from build123d import *

# Parameters (mm, degrees)
SKETCH3_W         = 2.032
SKETCH3_H         = 5.588
EXTRUDE1_DEPTH    = 2.088262662
CIRPATTERN1_COUNT = 6


with BuildPart() as part:
    # Sketch2 → Revolve1 (revolve)
    with BuildSketch(Plane.XY):
        Polygon((-4, 1.088262662), (-5.8419953, 0.40140039), (-7.003246048, 0.951561432), (-7.257246048, 0.951561432), (-7.3659953, 0.722019279), (-5.8419953, 0), (-4, 0.686862271), align=None)
    revolve(axis=Axis((0, 0, 0), (0, 1, 0)))

    # Sketch3 → Extrude1 (cut, through all)
    with BuildSketch(Plane(origin=(0, 0, 0), x_dir=(1, 0, 0), z_dir=(0, 1, 0))):
        with Locations((0, 2.794)):
            Rectangle(SKETCH3_W, SKETCH3_H)
    extrude1 = extrude(amount=EXTRUDE1_DEPTH, mode=Mode.SUBTRACT)

    # CirPattern1: Extrude1 ×6 about axis
    cirpattern1_axis = Axis((0, 0, 0), (0, 1, 0))
    for i in range(1, CIRPATTERN1_COUNT):
        add(extrude1.rotate(cirpattern1_axis, i * 360 / CIRPATTERN1_COUNT), mode=Mode.SUBTRACT)


solid = part.part
Design review of the part built by this model. Coordinates are the model's own, in mm. Coordinates: 2 decimals unless noted, no trailing zeros. Loops run counter-clockwise (first coordinate to the right, second up) from the corner with the lowest first, then second, coordinate; pieces in that order, holes last. Notation, with made-up numbers: M 85.25,30 L 116.25,30 A9 cw 116.25,41 Z; hole C 79.25,77 d1. An arc over 180 degrees is marked long. Use one line per item in the form item = value.
(1) Consider section C-C (x = 5). Give the number of separate pieces and of enclosed holes in the cut face, and give its area (3 significant figures).
Return value:
separate_pieces = 3
enclosed_holes = 0
area = 3.58 mm2
(2) Consider section A-A (z = 0). Write out the cut boundary in (x, y), and give its area (3 significant figures).
Return value:
outline = M -7.37,0.72 L -5.84,0 L -4,0.69 L -4,1.09 L -5.84,0.4 L -7,0.95 L -7.26,0.95 Z; M 4,0.69 L 5.84,0 L 7.37,0.72 L 7.26,0.95 L 7,0.95 L 5.84,0.4 L 4,1.09 Z
area = 2.61 mm2
(3) Consider section B-B (x = 0). Write out the cut boundary in (y, z).
Return value:
outline = M 0,-5.84 L 0.72,-7.37 L 0.95,-7.26 L 0.95,-7 L 0.4,-5.84 L 0.5,-5.59 L 0.09,-5.59 Z; M 0,5.84 L 0.09,5.59 L 0.5,5.59 L 0.4,5.84 L 0.95,7 L 0.95,7.26 L 0.72,7.37 Z
(4) Clearance check with flat-ended pins moving along their axes: P1, Ø1, axis at x = 4, z = 6, coming from the +Y side; P2, Ø3, axis at x = -2, z = -2, coming from the -Y side. State where each tip first meets the part, or that it passes through.
Return value:
P1 = 0.95
P2 = 0.56
(5) For line 1 along X through (y, z) = (0.65, -1.75); line 2 along X through (y, z) = (0.7, 2); line 3 along Y through (x, z) = (2.5, 5.5), list the stretches that pass through material, from the lowest coordinate up. Write a range as from..to.
Return value:
line_1 = -7..-6.12, 6.12..7
line_2 = -7.04..-6.16, 6.16..7.04
line_3 = 0.09..0.5
